Geometry check sheet. Reference: drawing and pictorial views, mm from the part's lowest x, y, z. A direction names the side the tool comes from. Round coordinates to 2 decimals unless told otherwise and drop trailing zeros. Write each loop counter-clockwise with the first axis right and the second up, starting at its lowest first coordinate (ties: lowest second). Pieces come first, ordered by that corner, then holes. Notation, with made-up numbers: M -18.5,-26 L -0.5,-26 A25 cw -0.5,10 Z; hole C -15.5,25.25 d3. An arc over 180 degrees is marked long. One line per item, written item: value. Start each with the question number.
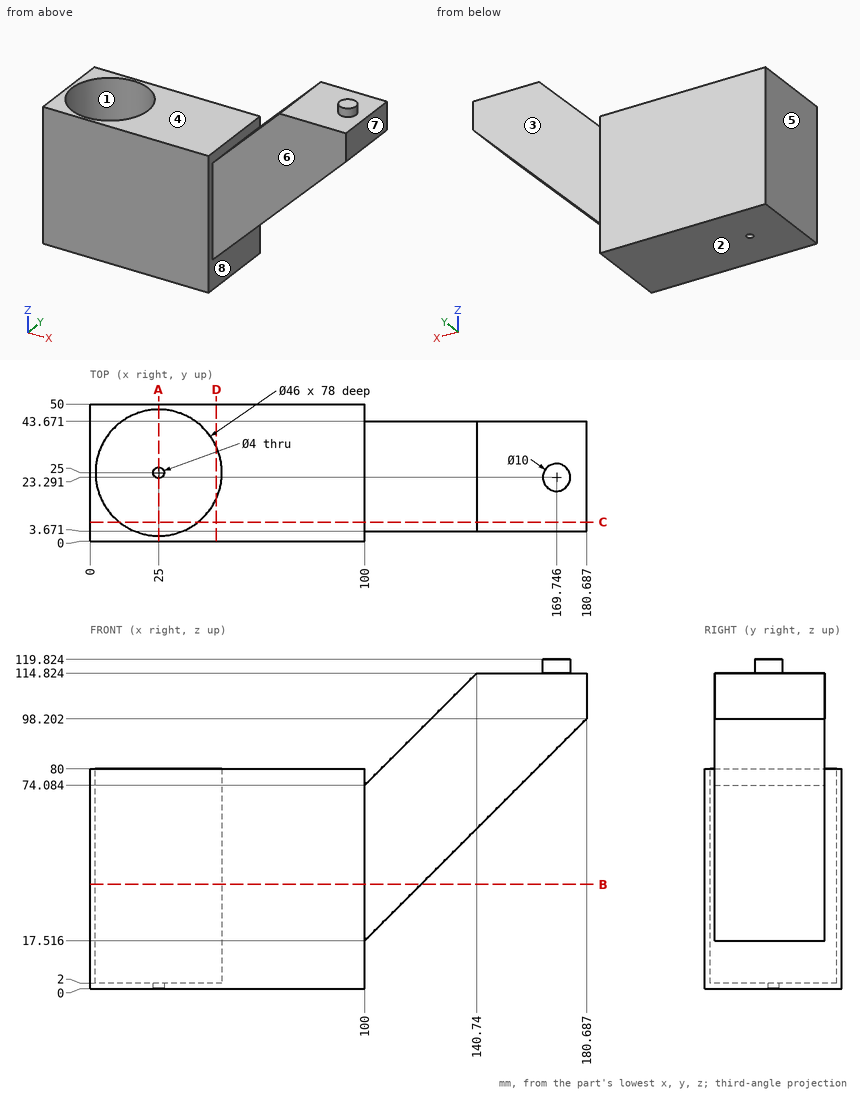
1) Access from +Z, -Z, +X, -X, +Y, -Y to the whole of each face (thin tool, end or side, straight path). Record for the marked faces 4, 5, 6, 7 and 8.
2) Cross-section at A-A (x = 25). Record the boundary of the cut face in (y, z), then the cut area to 3 significant figures.
3) Cross-section at C-C (y = 7). Record the boundary of the cut face in (x, z) (1 decimal).
4) Cross-section at B-B (z = 38). Record the boundary of the cut face in (x, y) (1 decimal), then the cut area to 3 significant figures.
5) Mould release check, pull along Y, two halves, no side actions. Record for the marked faces 1, 2 and 3: pulls with the +Y half, pulls with the -Y half, needs draft (parallel to the pull), parting line crosses it, or undercut.
6) Cross-section at D-D (x = 46). Record the boundary of the cut face in (y, z).
7) Thickness scan on line 1 (Y direction, x = 25, z = 55); line 2 (Z direction, x = 74, y = 12); line 3 (Z direction, x = 30, y = 43.5). Record the ranges inside material, lowest first.
8) Gauge pin test, flat ends, axial feed: pin 1 Ø1 at (x, y) = (160, 17) entering from -Z (1 decimal); pin 2 Ø25 at (y, z) = (27, 52) entering from +X (1 decimal); pin 3 Ø24 at (x, z) = (123.5, 58.5) entering from +Y; pin 4 Ø12 at (x, z) = (103.5, 30.5) entering from -Y. Record the tip position at first contact, or that the pin passes through.
Results below:
1. face 4: +Z, -X, +Y, -Y
1. face 5: +Z, -Z, -X, +Y, -Y
1. face 6: +Z, -Z, +X, -Y
1. face 7: +Z, -Z, +X, +Y, -Y
1. face 8: none
2. outline: M 0,0 L 23,0 L 23,2 L 2,2 L 2,80 L 0,80 Z; M 27,0 L 50,0 L 50,80 L 48,80 L 48,2 L 27,2 Z
2. area: 404 mm²
3. outline: M 0,0 L 100,0 L 100,17.5 L 180.7,98.2 L 180.7,114.8 L 140.7,114.8 L 100,74.1 L 100,80 L 39.3,80 L 39.3,2 L 10.7,2 L 10.7,80 L 0,80 Z
4. outline: M 0,0 L 100,0 L 100,3.7 L 120.5,3.7 L 120.5,43.7 L 100,43.7 L 100,50 L 0,50 Z; hole C 25,25 d46
4. area: 4,160 mm²
5. face 1: undercut
5. face 2: needs draft
5. face 3: pulls with the +Y half
6. outline: M 0,0 L 50,0 L 50,80 L 34.38,80 L 34.38,2 L 15.62,2 L 15.62,80 L 0,80 Z
7. line 1: y = 0 to 2, 48 to 50
7. line 2: z = 0 to 80
7. line 3: z = 0 to 2
8. pin 1: stops at z = 77
8. pin 2: stops at x = 147
8. pin 3: stops at y = 43.67
8. pin 4: stops at y = 0
